Geometry check sheet. Reference: the model listing, model coordinates, mm. A direction names the side the tool comes from. Round coordinates to 2 decimals unless told otherwise and drop trailing zeros. Order: outer loops, then holes, each group sorted by start corner. A loop starts at its lowest first (then second) coordinate and runs counter-clockwise, first axis right, second up. Notation, with made-up numbers: M 80.25,6.25 L 93.25,6.25 A11 cw 93.25,27.25 Z; hole C 64,-21.5 d1. An arc over 180 degrees is marked long. Return JSON: item names as keys, results as strings. Group by question number.
```python
from build123d import *

# Parameters (mm, degrees)
F0_W     = 82.55
F0_H     = 25.4
F0_R     = 3.175
F0_W_2   = 25.4
F0_H_2   = 82.55
F1_DEPTH = 2.794
F2_R     = 5.08


with BuildPart() as f1:
    # F0 (on Top) → F1 (new body)
    with BuildSketch(Plane.XY):
        Polygon((25.4, 114.3), (25.4, 31.75), (31.75, 31.75), (31.75, 25.4), (114.3, 25.4), align=None)
        with Locations((73.025, 12.7)):
            Rectangle(F0_W, F0_H)
        with Locations((44.45, 12.7)):
            Circle(F0_R, mode=Mode.SUBTRACT)
        with Locations((101.6, 12.7)):
            Circle(F0_R, mode=Mode.SUBTRACT)
        with Locations((12.7, 73.025)):
            Rectangle(F0_W_2, F0_H_2)
        with Locations((12.7, 44.45)):
            Circle(F0_R, mode=Mode.SUBTRACT)
        with Locations((12.7, 101.6)):
            Circle(F0_R, mode=Mode.SUBTRACT)
    extrude(amount=F1_DEPTH)

    # F2
    f2_edges = [f1.edges().sort_by_distance(p)[0] for p in [
        (31.75, 31.75, 1.397),
    ]]
    fillet(f2_edges, radius=F2_R)


solid = f1.part
```
Q1. Set-up check for faces 4 (the face through (13, 31.75, 1)), 5 (the face through (72, 0, 1)): record each of +Z, -Z, +X, -X, +Y, -Y from which the full face is reachable in a straight line by a thin tool's end or side.
Q2. Section check C-C on y = 101.6. Record the cut outline in (x, z) (3 decimals), plus the area to 3 significant figures.
Q3. Release check for a two-part mould opening along X. For faces 1 (the face through (44, 45, 0)), 2 (the face through (31.75, 14, 1)), 3 (the face through (12.3, 47.6, 1.4)) record: +X half, -X half, draft (parallel to the pull), parting line (faces both ways), or undercut.
Q4. Section check D-D on y = 12.7. Record the cut outline in (x, z) (3 decimals).
Q5. Material ranges on line 1 along Y through (x, z) = (12.7, 0.8) (3 decimals); line 2 along Y through (x, z) = (15.5, 1.05); line 3 along X through (y, z) = (14, 2), recorded low to high.
Q6. Section check A-A on z = 0.6. Record the cut outline in (x, y) (3 decimals).
Q7. Depth check by flat-ended pin: pin 1 Ø4 at (x, y) = (54.5, 42) entering from -Z; pin 2 Ø1.5 at (x, z) = (11.5, 1.5) entering from -Y. Enter the tip coordinate at first touch or a pass-through.
Q8. Section check B-B on x = 44.45. Record the cut outline in (y, z) (3 decimals), plus the area to 3 significant figures.
Geometry check:
{
 "1": {"face 4": "+Z, -Z, -X, -Y", "face 5": "+Z, -Z, +X, -X, -Y"},
 "2": {"outline": "M 0,0 L 9.525,0 L 9.525,2.794 L 0,2.794 Z; M 15.875,0 L 38.1,0 L 38.1,2.794 L 15.875,2.794 Z", "area": "88.7 mm^2"},
 "3": {"face 1": "draft", "face 2": "-X half", "face 3": "undercut"},
 "4": {"outline": "M 31.75,0 L 41.275,0 L 41.275,2.794 L 31.75,2.794 Z; M 47.625,0 L 98.425,0 L 98.425,2.794 L 47.625,2.794 Z; M 104.775,0 L 114.3,0 L 114.3,2.794 L 104.775,2.794 Z"},
 "5": {"line 1": "y = 31.75 to 41.275, 47.625 to 98.425, 104.775 to 114.3", "line 2": "y = 31.75 to 42.95, 45.95 to 100.1, 103.1 to 114.3", "line 3": "x = 31.75 to 41.55, 47.35 to 98.7, 104.5 to 114.3"},
 "6": {"outline": "M 0,31.75 L 26.67,31.75 A5.08 cw 31.75,26.67 L 31.75,0 L 114.3,0 L 114.3,25.4 L 25.4,114.3 L 0,114.3 Z; hole C 12.7,44.45 d6.35; hole C 12.7,101.6 d6.35; hole C 44.45,12.7 d6.35; hole C 101.6,12.7 d6.35"},
 "7": {"pin 1": "stops at z = 0", "pin 2": "stops at y = 31.75"},
 "8": {"outline": "M 0,0 L 9.525,0 L 9.525,2.794 L 0,2.794 Z; M 15.875,0 L 95.25,0 L 95.25,2.794 L 15.875,2.794 Z", "area": "248 mm^2"}
}
